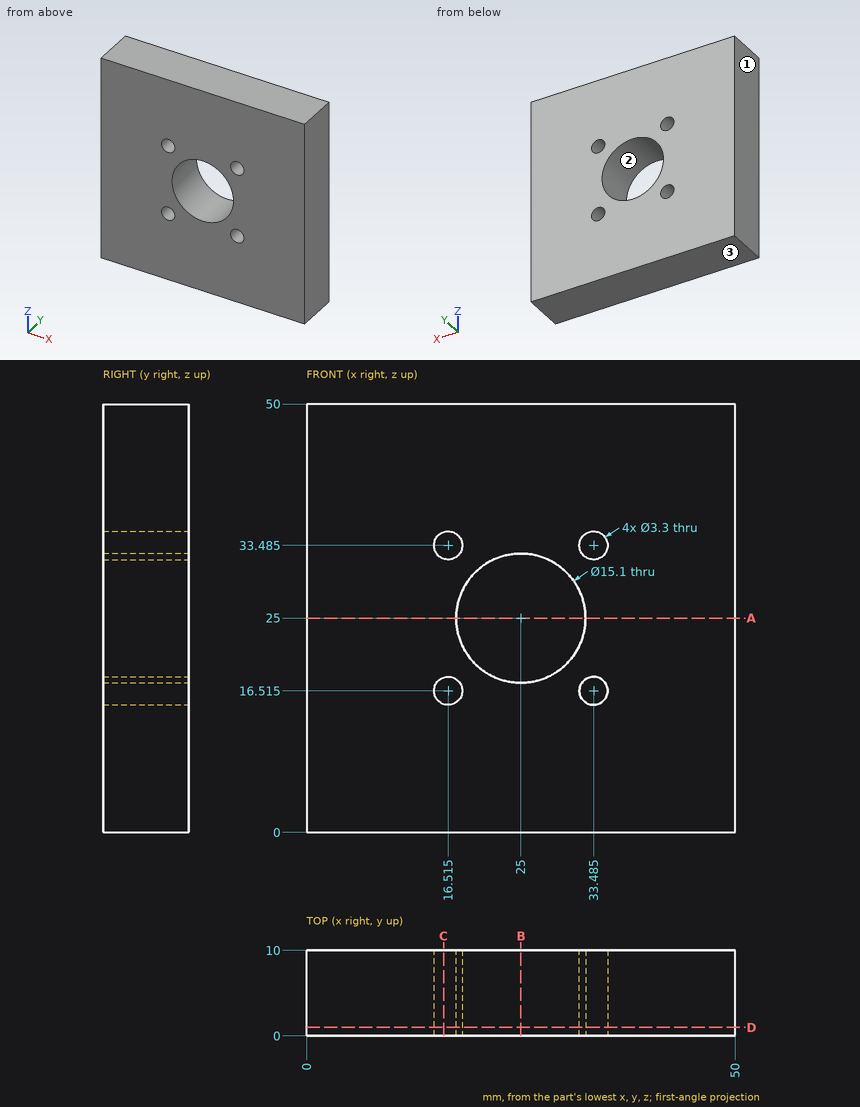
Study the drawing (mm; zero at the part's minimum x, y, z) and answer. Coordinates: 2 decimals unless noted, no trailing zeros. Write each loop counter-clockwise with the first axis right and the second up, starting at its lowest first coordinate (ties: lowest second). Pieces come first, ordered by that corner, then holes. Notation, with made-up numbers: (-27.5, 65.5) - (16.5, 65.5) arc R29 ccw to (16.5, 88.5) - close; hole circle Ø1 at (42.5, -17). An arc over 180 degrees is marked (long way). Answer as a JSON object with one key per item and string values. Group by question number.
1. A cutting plane is placed at A-A (z = 25). Determine the outline of the cut face in (x, y), plus the area to 3 significant figures.
2. A cutting plane is placed at C-C (x = 16). Determine the outline of the cut face in (y, z), plus the area to 3 significant figures.
3. The mould has two halves that part along Z. Classify the marked faces 1, 2 and 3: +Z half, -Z half, draft (parallel to the pull), parting line (faces both ways), or undercut.
4. A cutting plane is placed at D-D (y = 1). Give the number of separate pieces and of enclosed holes in the cut face, plus the area to 3 significant figures.
5. Consider L1, parallel to Z at x = 33.5, y = 5.25 (1 decimal); L2, parallel to X at y = 6, z = 25; L3, parallel to X at y = 2, z = 35. Determine where each line is inside the solid, lowest interval first. Write a range as [from, to].
6. This flat-tipped pin is pushed along its axis until it touches: P1, Ø2.5, axis at x = 33.49, z = 16.51, coming from the +Y side. Where does it stop, or does it pass through?
7. A cutting plane is placed at B-B (x = 25). Determine the outline of the cut face in (y, z), plus the area to 3 significant figures.
Worked out:
{
 "1": {"outline": "(0, 0) - (17.45, 0) - (17.45, 10) - (0, 10) - close; (32.55, 0) - (50, 0) - (50, 10) - (32.55, 10) - close", "area": "349 mm²"},
 "2": {"outline": "(0, 0) - (10, 0) - (10, 14.95) - (0, 14.95) - close; (0, 18.08) - (10, 18.08) - (10, 31.92) - (0, 31.92) - close; (0, 35.05) - (10, 35.05) - (10, 50) - (0, 50) - close", "area": "437 mm²"},
 "3": {"face 1": "draft", "face 2": "undercut", "face 3": "-Z half"},
 "4": {"separate pieces": "1", "enclosed holes": "5", "area": "2,290 mm²"},
 "5": {"L1": "z = [0, 14.9], [18.2, 31.8], [35.1, 50]", "L2": "x = [0, 17.45], [32.55, 50]", "L3": "x = [0, 15.86], [17.17, 32.83], [34.14, 50]"},
 "6": {"P1": "passes through"},
 "7": {"outline": "(0, 0) - (10, 0) - (10, 17.45) - (0, 17.45) - close; (0, 32.55) - (10, 32.55) - (10, 50) - (0, 50) - close", "area": "349 mm²"}
}
